Design review of the part shown in the three views and the two pictorial views. Dimensions are in mm from the part's minimum x, y and z. Round coordinates to 2 decimals unless told otherwise and drop trailing zeros. Order: outer loops, then holes, each group sorted by start corner. A loop starts at its lowest first (then second) coordinate and runs counter-clockwise, first axis right, second up. Notation, with made-up numbers: M -28.75,81.25 L -15.75,81.25 A31 ccw -15.75,114.25 Z; hole C -7,-2 d4. An arc over 180 degrees is marked long. Use a Markdown table: item, result. Add a question column.
(1) Take a section at B-B (z = 2.2). Write out the cut boundary in (x, y).
(2) Take a section at A-A (y = 20.5). Write out the cut boundary in (x, z).
(3) Take a section at C-C (x = 23.5). Write out the cut boundary in (y, z).
(4) The part is to be moulded in two halves that separate along X. For the marked faces 1 and 2, say which applies: released by +X, released by -X, zero draft, split by the parting line, or undercut.
(5) For pin 1 (1.5 mm diameter, centred on x = 47, y = 64, fed in from +Z), flat-tipped, find the tip position at first contact; note if it passes through.
(6) To check wall thickness, follow probe 1 along Y at (x, z) = (32, 4.75); probe 2 along X at (y, z) = (55.5, 1.45); probe 3 along Z at (x, y) = (49, 12.5). State the ranges of each line that lie inside material, in increasing order. Write a range as from..to.
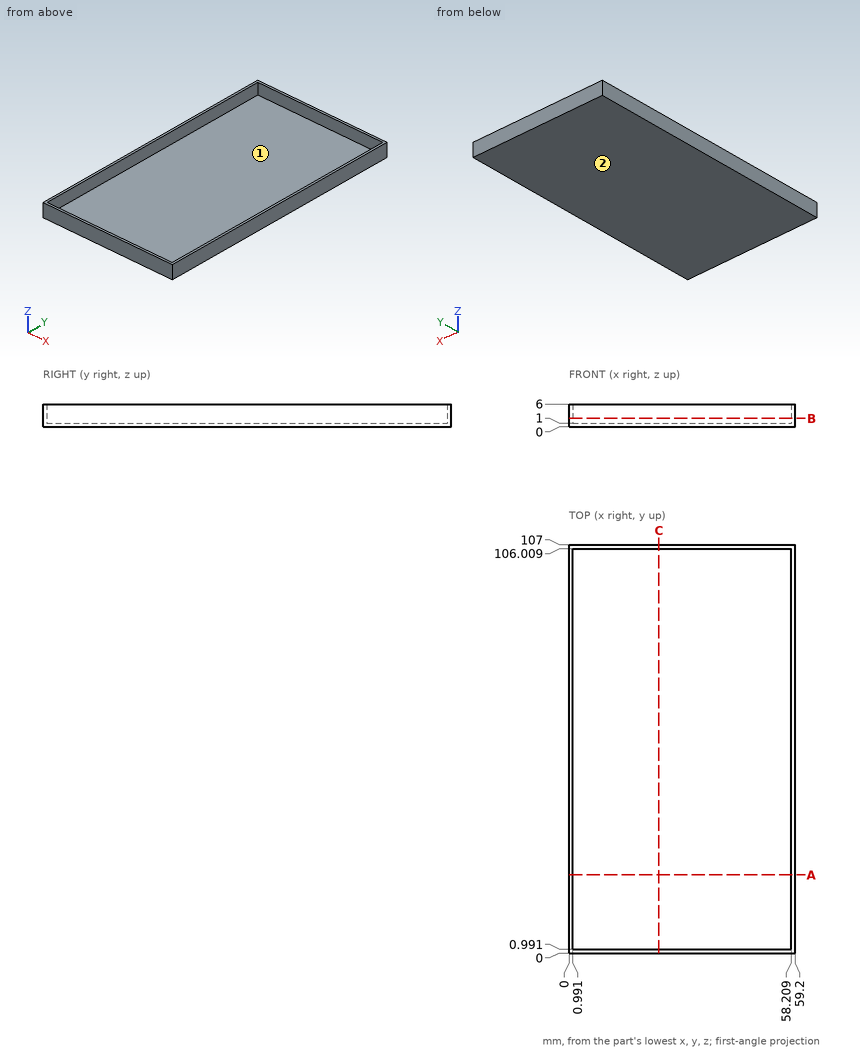
Verdict:
| question | item | result |
|---|---|---|
| 1 | outline | M 0,0 L 59.2,0 L 59.2,107 L 0,107 Z; hole M 0.99,0.99 L 58.21,0.99 L 58.21,106.01 L 0.99,106.01 Z |
| 2 | outline | M 0,0 L 59.2,0 L 59.2,6 L 58.21,6 L 58.21,1 L 0.99,1 L 0.99,6 L 0,6 Z |
| 3 | outline | M 0,0 L 107,0 L 107,6 L 106.01,6 L 106.01,1 L 0.99,1 L 0.99,6 L 0,6 Z |
| 4 | face 1 | undercut |
| 4 | face 2 | zero draft |
| 5 | pin 1 | stops at z = 1 |
| 6 | probe 1 | y = 0..0.99, 106.01..107 |
| 6 | probe 2 | x = 0..0.99, 58.21..59.2 |
| 6 | probe 3 | z = 0..1 |
